Source: CAD feature listing. Evaluate the final solid. Frame: model axes, mm. A direction names the side the tool comes from. Coordinates: 2 decimals unless noted, no trailing zeros. Order: outer loops, then holes, each group sorted by start corner. A loop starts at its lowest first (then second) coordinate and runs counter-clockwise, first axis right, second up.
```python
from build123d import *

# Parameters (mm, degrees)
SKETCH2_W           = 56
SKETCH2_H           = 55
BOSS_EXTRUDE1_DEPTH = 5
SKETCH4_R           = 11.5
CUT_EXTRUDE1_DEPTH  = 3
SKETCH5_R           = 1.75
CUT_EXTRUDE3_DEPTH  = 54
SKETCH6_W           = 56
SKETCH6_H           = 55
SKETCH6_W_2         = 46
SKETCH6_H_2         = 45
BOSS_EXTRUDE2_DEPTH = 5
SKETCH3_R           = 2.75
SKETCH3_R_2         = 1.75
CUT_EXTRUDE2_DEPTH  = 12
SKETCH5_2_R         = 1.75
CUT_EXTRUDE4_DEPTH  = 33
SKETCH7_R           = 2.75
CUT_EXTRUDE5_DEPTH  = 4


with BuildPart() as part:
    # Sketch2 → Boss-Extrude1 (new body)
    with BuildSketch(Plane(origin=(0, 0, 0), x_dir=(1, 0, 0), z_dir=(0, 1, 0))):
        Rectangle(SKETCH2_W, SKETCH2_H)
    extrude(amount=BOSS_EXTRUDE1_DEPTH)

    # Sketch4 → Cut-Extrude1 (cut)
    with BuildSketch(Plane.XZ):
        Circle(SKETCH4_R)
    extrude(amount=-CUT_EXTRUDE1_DEPTH, mode=Mode.SUBTRACT)

    # Sketch5 → Cut-Extrude3 (cut)
    with BuildSketch(Plane(origin=(0, 5, 0), x_dir=(1, 0, 0), z_dir=(0, 1, 0))):
        with Locations((-25.5, 17.5)):
            Circle(SKETCH5_R)
        with Locations((25.5, -17.5)):
            Circle(SKETCH5_R)
        with Locations((-25.5, -17.5)):
            Circle(SKETCH5_R)
        with Locations((25.5, 17.5)):
            Circle(SKETCH5_R)
    extrude(amount=-CUT_EXTRUDE3_DEPTH, mode=Mode.SUBTRACT)

    # Sketch6 → Boss-Extrude2 (add)
    with BuildSketch(Plane.XZ):
        Rectangle(SKETCH6_W, SKETCH6_H)
        Rectangle(SKETCH6_W_2, SKETCH6_H_2, mode=Mode.SUBTRACT)
    extrude(amount=BOSS_EXTRUDE2_DEPTH)

    # Sketch3 → Cut-Extrude2 (cut)
    with BuildSketch(Plane(origin=(0, 5, 0), x_dir=(1, 0, 0), z_dir=(0, 1, 0))):
        Circle(SKETCH3_R)
        with Locations((-15.5, 15.5)):
            Circle(SKETCH3_R_2)
        with Locations((15.5, 15.5)):
            Circle(SKETCH3_R_2)
        with Locations((15.5, -15.5)):
            Circle(SKETCH3_R_2)
        with Locations((-15.5, -15.5)):
            Circle(SKETCH3_R_2)
    extrude(amount=-CUT_EXTRUDE2_DEPTH, mode=Mode.SUBTRACT)

    # Sketch5<2> → Cut-Extrude4 (cut)
    with BuildSketch(Plane(origin=(0, 5, 0), x_dir=(1, 0, 0), z_dir=(0, 1, 0))):
        with Locations((-25.5, 17.5)):
            Circle(SKETCH5_2_R)
        with Locations((25.5, -17.5)):
            Circle(SKETCH5_2_R)
        with Locations((-25.5, -17.5)):
            Circle(SKETCH5_2_R)
        with Locations((25.5, 17.5)):
            Circle(SKETCH5_2_R)
    extrude(amount=-CUT_EXTRUDE4_DEPTH, mode=Mode.SUBTRACT)

    # Sketch7 → Cut-Extrude5 (cut)
    with BuildSketch(Plane(origin=(0, 5, 0), x_dir=(1, 0, 0), z_dir=(0, 1, 0))):
        with Locations((-15.5, 15.5)):
            Circle(SKETCH7_R)
        with Locations((15.5, 15.5)):
            Circle(SKETCH7_R)
        with Locations((15.5, -15.5)):
            Circle(SKETCH7_R)
        with Locations((-15.5, -15.5)):
            Circle(SKETCH7_R)
        with Locations((-25.5, 17.5)):
            Circle(SKETCH7_R)
        with Locations((-25.5, -17.5)):
            Circle(SKETCH7_R)
        with Locations((25.5, 17.5)):
            Circle(SKETCH7_R)
        with Locations((25.5, -17.5)):
            Circle(SKETCH7_R)
    extrude(amount=-CUT_EXTRUDE5_DEPTH, mode=Mode.SUBTRACT)


solid = part.part
```
Q1. Material intervals for line 1 along Z through (x, y) = (-25.5, 1.85); line 2 along Z through (x, y) = (-25.5, -2.05); line 3 along Z through (x, y) = (-7.5, -4.25), sorted ascending.
Solutions:
line 1: z = -27.5 to -20.25, -14.75 to 14.75, 20.25 to 27.5
line 2: z = -27.5 to -19.25, -15.75 to 15.75, 19.25 to 27.5
line 3: z = -27.5 to -22.5, 22.5 to 27.5
Q2. Section query C-C on x = 0. Output: boundary loops of the cut face in (y, z).
Solutions:
outline: (-5, -27.5) - (5, -27.5) - (5, -2.75) - (3, -2.75) - (3, -11.5) - (0, -11.5) - (0, -22.5) - (-5, -22.5) - close; (-5, 22.5) - (0, 22.5) - (0, 11.5) - (3, 11.5) - (3, 2.75) - (5, 2.75) - (5, 27.5) - (-5, 27.5) - close
Q3. Set-up query: faces 4 (the cylindrical face through (-18.247, 3.028, 15.379)), 5 (the flat face through (0, 5, -6)), 6 (the flat face through (-5.43, 0, -10.31)). Return all of +Z, -Z, +X, -X, +Y, -Y with unobstructed straight access to the full face (end or side cutting, diameter ignored); none if empty.
Solutions:
face 4: +Y
face 5: +Z, -Z, +X, -X, +Y
face 6: -Y
Q4. Section query A-A on x = 15.5. Output: boundary loops of the cut face in (y, z).
Solutions:
outline: (-5, -27.5) - (5, -27.5) - (5, -18.25) - (1, -18.25) - (1, -17.25) - (0, -17.25) - (0, -22.5) - (-5, -22.5) - close; (-5, 22.5) - (0, 22.5) - (0, 17.25) - (1, 17.25) - (1, 18.25) - (5, 18.25) - (5, 27.5) - (-5, 27.5) - close; (0, -13.75) - (1, -13.75) - (1, -12.75) - (5, -12.75) - (5, 12.75) - (1, 12.75) - (1, 13.75) - (0, 13.75) - close
Q5. Section query B-B on y = -2.5. Output: boundary loops of the cut face in (x, z).
Solutions:
outline: (-28, -27.5) - (28, -27.5) - (28, 27.5) - (-28, 27.5) - close; hole circle Ø3.5 at (-25.5, -17.5); hole circle Ø3.5 at (-25.5, 17.5); hole (-23, -22.5) - (23, -22.5) - (23, 22.5) - (-23, 22.5) - close; hole circle Ø3.5 at (25.5, -17.5); hole circle Ø3.5 at (25.5, 17.5)
Q6. Section query D-D on z = -1. Output: boundary loops of the cut face in (x, y).
Solutions:
outline: (-28, -5) - (-23, -5) - (-23, 0) - (-11.46, 0) - (-11.46, 3) - (-2.56, 3) - (-2.56, 5) - (-28, 5) - close; (2.56, 3) - (11.46, 3) - (11.46, 0) - (23, 0) - (23, -5) - (28, -5) - (28, 5) - (2.56, 5) - close
Q7. Pin query (flat end, axial travel): P1, Ø4, axis at x = 25.5, z = -17.5, coming from the +Y side; P2, Ø4.5, axis at x = -15.5, z = 15.5, coming from the -Y side. Return the tip coordinate at first contact, or that it passes through.
Solutions:
P1: stops at y = 1
P2: stops at y = 0
Q8. Pull-direction query (Z, two-part tool) for faces 1 (the flat face through (0, 0, -27.5)), 2 (the flat face through (0, 0, 27.5)), 3 (the cylindrical face through (24.21, -1.96, 16.32)); classes: pulls with the +Z half, pulls with the -Z half, needs draft (parallel to the pull), parting line crosses it, or undercut.
Solutions:
face 1: pulls with the -Z half
face 2: pulls with the +Z half
face 3: undercut
